Here's how the part is built. I have some questions about the finished solid (model axes, mm). Face numbers are marked on the shaded views. A direction names the side the tool comes from. Coordinates: 2 decimals unless noted, no trailing zeros. Order: outer loops, then holes, each group sorted by start corner. A loop starts at its lowest first (then second) coordinate and runs counter-clockwise, first axis right, second up. Notation, with made-up numbers: (-34.75, 72.25) - (-28.75, 72.25) arc R15 cw to (-28.75, 94.25) - close; hole circle Ø11 at (63.5, -12.5). An arc over 180 degrees is marked (long way). Answer as CSV lines item,"result". Start each with the question number.
Item 1: I need wall thicknesses on line 1 (Y direction, x = 42, z = 60.5); line 2 (Z direction, x = 6.5, y = 5); line 3 (X direction, y = 32, z = 57). Which ranges of each line are inside material? Lowest first, please.
Item 2: We'd pull the mould along X, two halves only. Please class the marked faces 1, 2, 3 and 4: pulls with the +X half, pulls with the -X half, needs draft (parallel to the pull), parting line crosses it, or undercut.
Item 3: Imagine slicing it at C-C on z = 60.5. List the corners of the cut face in (x, y) for me, and give its area (3 significant figures).
Item 4: Imagine slicing it at A-A on x = 27. List the corners of the cut face in (y, z) for me, and give its area (3 significant figures).
Item 5: Imagine slicing it at B-B on y = 29. List the corners of the cut face in (x, z) for me.
Item 6: On a 3-axis mill with a long thin cutter (end or side, diameter ignored), from which of +Z, -Z, +X, -X, +Y, -Y can I reach the whole of each face in a straight line? I mean the marked faces 5 and 6. Say none if no direction works.
Item 7: I'm going to push flat-ended pins straight in: pin 1 (17 mm diameter, centred on y = 29, z = 63, fed in from -X); pin 2 (1.5 mm diameter, centred on x = 48.5, y = 43, fed in from +Z). Where does each tip first touch, or does it pass through?
from build123d import *

# Parameters (mm, degrees)
SKETCH1_W           = 61
SKETCH1_H           = 50
SKETCH1_W_2         = 53
SKETCH1_H_2         = 42
BOSS_EXTRUDE1_DEPTH = 70.6
SKETCH2_W           = 61
SKETCH2_H           = 50
BOSS_EXTRUDE2_DEPTH = 49.6
SKETCH3_R           = 19
CUT_EXTRUDE1_DEPTH  = 10


with BuildPart() as part:
    # Sketch1 → Boss-Extrude1 (new body)
    with BuildSketch(Plane.XY):
        with Locations((30.5, 25)):
            Rectangle(SKETCH1_W, SKETCH1_H)
        with Locations((30.5, 25)):
            Rectangle(SKETCH1_W_2, SKETCH1_H_2, mode=Mode.SUBTRACT)
    extrude(amount=BOSS_EXTRUDE1_DEPTH)

    # Sketch2 → Boss-Extrude2 (add)
    with BuildSketch(Plane(origin=(0, 0, 0), x_dir=(-1, 0, 0), z_dir=(0, 0, -1))):
        with Locations((-30.5, 25)):
            Rectangle(SKETCH2_W, SKETCH2_H)
    extrude(amount=-BOSS_EXTRUDE2_DEPTH)

    # Sketch3 → Cut-Extrude1 (cut)
    with BuildSketch(Plane(origin=(61, 0, 0), x_dir=(0, 0, -1), z_dir=(1, 0, 0))):
        with Locations((-70.6, 25)):
            Circle(SKETCH3_R)
    extrude(amount=-CUT_EXTRUDE1_DEPTH, mode=Mode.SUBTRACT)


solid = part.part
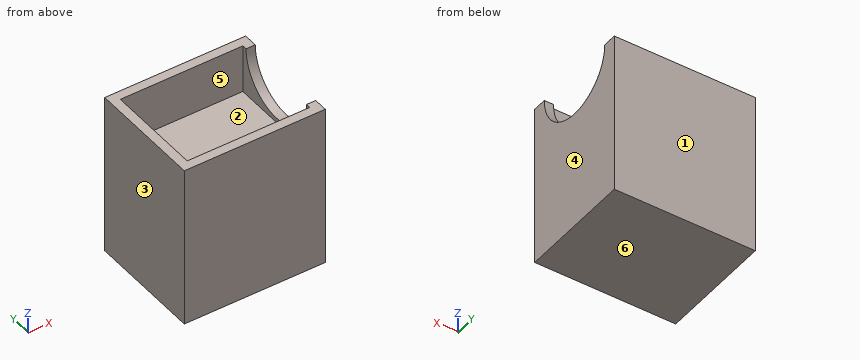
Responses:
1,line 1,"y = 0 to 4, 46 to 50"
1,line 2,"z = 0 to 49.6"
1,line 3,"x = 0 to 4"
2,face 1,"needs draft"
2,face 2,"undercut"
2,face 3,"pulls with the -X half"
2,face 4,"pulls with the +X half"
3,outline,"(0, 0) - (61, 0) - (61, 8.91) - (57, 8.91) - (57, 4) - (4, 4) - (4, 46) - (57, 46) - (57, 41.09) - (61, 41.09) - (61, 50) - (0, 50) - close"
3,area,"695 mm^2"
4,outline,"(0, 0) - (50, 0) - (50, 70.6) - (46, 70.6) - (46, 49.6) - (4, 49.6) - (4, 70.6) - (0, 70.6) - close"
4,area,"2,650 mm^2"
5,outline,"(0, 0) - (61, 0) - (61, 52.03) - (57, 52.03) - (57, 49.6) - (4, 49.6) - (4, 70.6) - (0, 70.6) - close"
6,face 5,"+Z"
6,face 6,"-Z, +X, -X, +Y, -Y"
7,pin 1,"stops at x = 0"
7,pin 2,"stops at z = 49.6"
